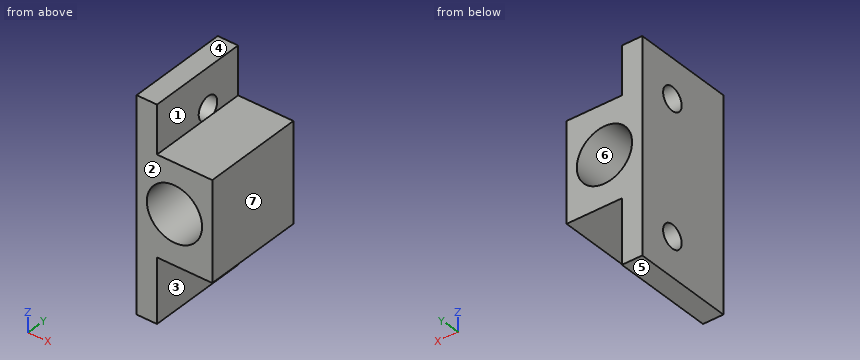
Autodesk Inventor part; units mm, degrees
ref_plane "YZ Plane" through (0, 0, 0) normal (1, 0, 0) x (0, 1, 0)
ref_plane "XZ Plane" through (0, 0, 0) normal (0, 1, 0) x (-1, 0, 0)
ref_plane "XY Plane" through (0, 0, 0) normal (0, 0, 1) x (1, 0, 0)
sketch "Sketch1" plane through (0, 0, 0) normal (0, 1, 0) x (-1, 0, 0)
  line L0 (26, -72.5) -> (-26, -72.5)
  line L1 (-26, -72.5) -> (-26, 72.5)
  line L2 (-26, 72.5) -> (26, 72.5)
  line L3 (26, 72.5) -> (26, -72.5)
  line L4 (26, -72.5) -> (-26, 72.5) construction
  line L5 (-26, -72.5) -> (26, 72.5) construction
  point P0 (0, 0)
  dimension "d0" = 52
  dimension "d1" = 145
extrude "Extrusion1" add sketch "Sketch1" along normal mid plane 70
sketch "Sketch2" plane through (0, 35, 0) normal (0, 1, 0) x (1, 0, 0)
  line L0 (26, -72.5) -> (26, 72.5)
  line L1 (26, 72.5) -> (-12, 72.5)
  line L2 (26, 72.5) -> (-26, 72.5)
  line L3 (-12, 72.5) -> (-12, 28.5)
  line L4 (-12, 28.5) -> (26, 28.5)
  line L5 (26, 28.5) -> (26, -39.5)
  line L6 (-26, -72.5) -> (26, -72.5)
  line L7 (26, -39.5) -> (-12, -39.5)
  line L8 (-12, -39.5) -> (-12, -72.5)
  point P0 (0, 0)
  point P1 (-12, -37.5)
  dimension "d4" = 38
  dimension "d5" = 44
  dimension "d6" = 68
extrude "Extrusion2" cut sketch "Sketch2" against normal blind 70
sketch "Sketch3" plane through (-12, 35, 72.5) normal (1, 0, 0) x (0, 0, -1)
  line L0 (145, 0) -> (0, 0)
  line L1 (0, 0) -> (0, -26)
  line L2 (0, 0) -> (0, -70)
  line L3 (0, -26) -> (27, -26)
  circle A0 centre (27, -26) radius 8
  line L4 (145, 0) -> (145, -26)
  line L5 (145, 0) -> (145, -70)
  line L6 (145, -26) -> (118, -26)
  circle A1 centre (118, -26) radius 8
  point P0 (72.5, -35)
  dimension "d9" = 26
  dimension "d10" = 27
  dimension "d11" = 16
  dimension "d12" = 26
  dimension "d13" = 27
  dimension "d14" = 16
extrude "Extrusion3" cut sketch "Sketch3" against normal blind 70
sketch "Sketch4" plane through (0, 35, 0) normal (0, 1, 0) x (1, 0, 0)
  line L0 (26, 28.5) -> (26, -39.5)
  line L1 (26, -39.5) -> (0, -39.5)
  line L2 (0, -39.5) -> (0, -5.5)
  circle A0 centre (0, -5.5) radius 19
  point P0 (0, 0)
  dimension "d17" = 34
  dimension "d18" = 38
extrude "Extrusion4" cut sketch "Sketch4" against normal blind 70
properties part number "carriage"
The model under review builds one solid part; all positions refer to its coordinate system, in mm. Face numbers are marked on the shaded views. A direction names the side the tool comes from. Give positions to 0.01 mm unless a question says otherwise; leave off trailing zeros. Order: outer loops, then holes, each group sorted by start corner. A loop starts at its lowest first (then second) coordinate and runs counter-clockwise, first axis right, second up. Notation, with made-up numbers: M 83.25,69.5 L 110.25,69.5 A22 ccw 110.25,79.5 Z; hole C -32,7 d9. An arc over 180 degrees is marked long. Use one line per item in the form item = value. Start each with the question number.
Item 1: The part is to be moulded in two halves that separate along Z. For the marked faces 4, 5, 6 and 7, say which applies: pulls with the +Z half, pulls with the -Z half, needs draft (parallel to the pull), parting line crosses it, or undercut.
Item 2: Insertion check: pin 1 Ø2 at (y, z) = (-17, -52.5) entering from +X; pin 2 Ø14.5 at (y, z) = (9, -45.5) entering from -X; pin 3 Ø6 at (x, y) = (-6.5, 18.5) entering from +Z. Each pin has a flat end and moves straight along its axis. Give the tip position at first contact, or say it passes through.
Item 3: We need section A-A on z = 5.5. Give the boundary of the cut face in (x, y).
Item 4: To check wall thickness, follow line 1 along Z through (x, y) = (0, -14.5); line 2 along Z through (x, y) = (-20.5, 8.5); line 3 along Z through (x, y) = (-21.5, 5). State the ranges of each line that lie inside material, in increasing order. Write a range as from..to.
Item 5: We need section B-B on x = 0. Give the boundary of the cut face in (y, z).
Item 6: We need section C-C on y = 23.5. Give the boundary of the cut face in (x, z).
Item 7: We need section D-D on x = -16. Give the boundary of the cut face in (y, z), plus the area to 3 significant figures.
Item 8: For the marked faces 1, 2 and 3, list the 3-axis set-ups (+Z, -Z, +X, -X, +Y, -Y) from which the entire face can be reached by the end or side of a thin tool; tool diameter is ignored.
Completed:
q1.face_4 = pulls with the +Z half
q1.face_5 = pulls with the -Z half
q1.face_6 = undercut
q1.face_7 = needs draft
q2.pin_1 = -12
q2.pin_2 = through
q2.pin_3 = 39.5
q3.outline = M -26,-35 L -19,-35 L -19,35 L -26,35 Z; M 19,-35 L 26,-35 L 26,35 L 19,35 Z
q4.line_1 = -28.5..-13.5, 24.5..39.5
q4.line_2 = -72.5..-53.48, -37.52..37.52, 53.48..72.5
q4.line_3 = -72.5..-52.43, -38.57..38.57, 52.43..72.5
q5.outline = M -35,-28.5 L 35,-28.5 L 35,-13.5 L -35,-13.5 Z; M -35,24.5 L 35,24.5 L 35,39.5 L -35,39.5 Z
q6.outline = M -26,-72.5 L -12,-72.5 L -12,-28.5 L 26,-28.5 L 26,39.5 L -12,39.5 L -12,72.5 L -26,72.5 Z; hole C 0,5.5 d38
q7.outline = M -35,-72.5 L 35,-72.5 L 35,-4.75 L -35,-4.75 Z; M -35,15.75 L 35,15.75 L 35,72.5 L -35,72.5 Z; hole C 9,-45.5 d16; hole C 9,45.5 d16
q7.area = 8,310 mm²
q8.face_1 = +Z, +X, +Y, -Y
q8.face_2 = +Z, -Z, +X, -X, -Y
q8.face_3 = -Z, +X, +Y, -Y
